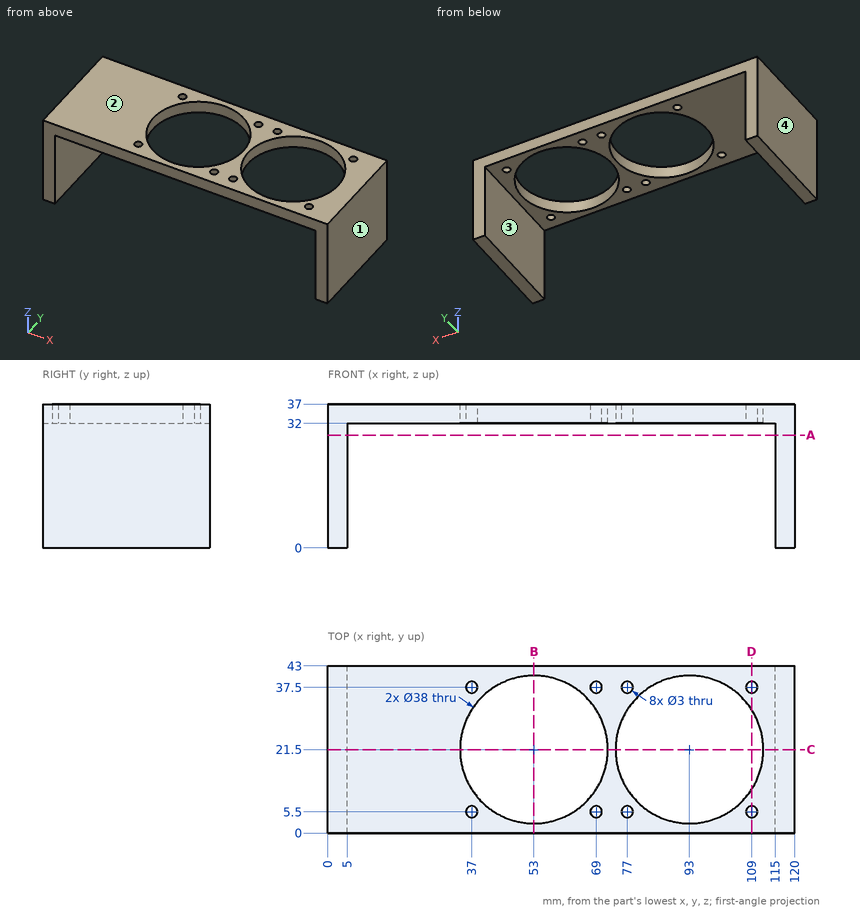
Study the drawing (mm; zero at the part's minimum x, y, z) and answer. Give positions to 0.01 mm unless a question says otherwise; leave off trailing zeros. Loops run counter-clockwise (first coordinate to the right, second up) from the corner with the lowest first, then second, coordinate; pieces in that order, holes last. Notation, with made-up numbers: M 41,66 L 91,66 A7 cw 91,78 Z; hole C 57.5,51.25 d4. An arc over 180 degrees is marked long. One line per item, written item: value. Start each with the question number.
1. Determine the mould class of the marked faces 1, 2, 3 and 4 for opening direction X: released by +X, released by -X, zero draft, split by the parting line, or undercut.
2. Find section D-D (x = 109). Give the vertices of the cut face in (y, z).
3. Find section A-A (z = 29). Give the vertices of the cut face in (x, y), and give its area (3 significant figures).
4. Find the intervals of material crossed by probe 1 along X at (y, z) = (11.5, 18); probe 2 along Y at (x, z) = (109, 33.9); probe 3 along Z at (x, y) = (114, 25), in increasing order.
5. Find section C-C (y = 21.5). Give the vertices of the cut face in (x, z), and give its area (3 significant figures).
6. Find section B-B (x = 53). Give the vertices of the cut face in (y, z).
7. This flat-tipped pin is pushed along its axis until it touches: P1, Ø6, axis at x = 68.5, y = 10.5, coming from the -Z side. Where does it stop, or does it pass through?
Reported:
1. face 1: released by +X
1. face 2: zero draft
1. face 3: undercut
1. face 4: released by -X
2. outline: M 0,32 L 4,32 L 4,37 L 0,37 Z; M 7,32 L 11.25,32 L 11.25,37 L 7,37 Z; M 31.75,32 L 36,32 L 36,37 L 31.75,37 Z; M 39,32 L 43,32 L 43,37 L 39,37 Z
3. outline: M 0,0 L 5,0 L 5,43 L 0,43 Z; M 115,0 L 120,0 L 120,43 L 115,43 Z
3. area: 430 mm²
4. probe 1: x = 0 to 5, 115 to 120
4. probe 2: y = 0 to 4, 7 to 11.25, 31.75 to 36, 39 to 43
4. probe 3: z = 32 to 37
5. outline: M 0,0 L 5,0 L 5,32 L 34,32 L 34,37 L 0,37 Z; M 72,32 L 74,32 L 74,37 L 72,37 Z; M 112,32 L 115,32 L 115,0 L 120,0 L 120,37 L 112,37 Z
5. area: 540 mm²
6. outline: M 0,32 L 2.5,32 L 2.5,37 L 0,37 Z; M 40.5,32 L 43,32 L 43,37 L 40.5,37 Z
7. P1: stops at z = 32
